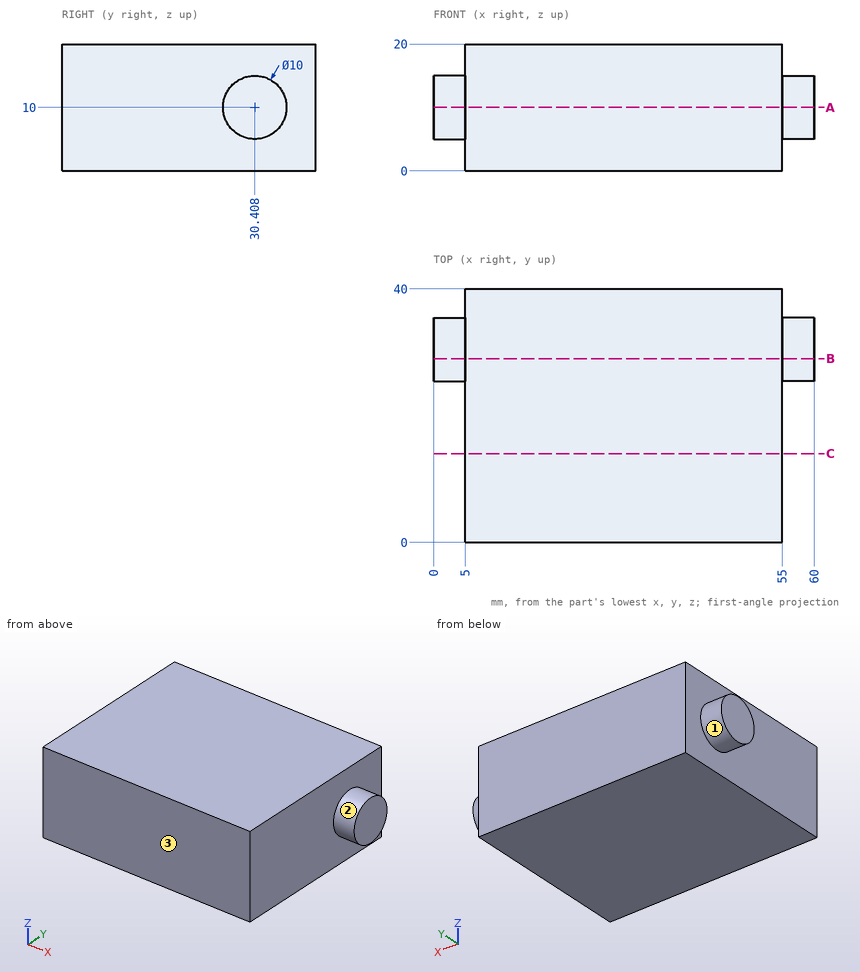
Job drawing, mm, ordinate dimensions from the low corner. One solid piece. A direction names the side the tool comes from. Coordinates: 2 decimals unless noted, no trailing zeros. Write each loop counter-clockwise with the first axis right and the second up, starting at its lowest first coordinate (ties: lowest second). Pieces come first, ordered by that corner, then holes. Notation, with made-up numbers: M 13,52.25 L 63,52.25 A24 cw 63,83.25 Z; hole C -5,-32.75 d9. An arc over 180 degrees is marked long. Answer as a JSON object with one key per item and string values. Group by question number.
1) Saw through at C-C (y = 14). Write the cut outline in (x, z), plus the area to 3 significant figures.
2) Saw through at B-B (y = 29). Write the cut outline in (x, z), plus the area to 3 significant figures.
3) Wall check: line 1 (X direction, y = 28, z = 18.75); line 2 (Z direction, x = 57, y = 35) (1 decimal); line 3 (Y direction, x = 56.5, z = 6.5). Give the ranges that are in metal, low to high. Write a range as from..to.
4) Saw through at A-A (z = 10). Write the cut outline in (x, y).
5) Pin check, flat tip, straight feed: pin 1 Ø1 at (y, z) = (23.5, 2.5) entering from -X. Stop position of the tip, or through.
6) Tool access for the marked faces 1, 2 and 3: list every direction of +Z, -Z, +X, -X, +Y, -Y with a clear straight run to the whole face (end or side of a thin tool).
Values follow:
{
 "1": {"outline": "M 5,0 L 55,0 L 55,20 L 5,20 Z", "area": "1,000 mm2"},
 "2": {"outline": "M 0,5.2 L 5,5.2 L 5,0 L 55,0 L 55,5.2 L 60,5.2 L 60,14.8 L 55,14.8 L 55,20 L 5,20 L 5,14.8 L 0,14.8 Z", "area": "1,100 mm2"},
 "3": {"line 1": "x = 5..55", "line 2": "z = 8..12", "line 3": "y = 26.84..33.98"},
 "4": {"outline": "M 0,25.41 L 5,25.41 L 5,0 L 55,0 L 55,25.41 L 60,25.41 L 60,35.41 L 55,35.41 L 55,40 L 5,40 L 5,35.41 L 0,35.41 Z"},
 "5": {"pin 1": "stops at x = 5"},
 "6": {"face 1": "-X", "face 2": "+X", "face 3": "+Z, -Z, +X, -X, -Y"}
}
